from build123d import *

# Parameters (mm, degrees)
F1_DEPTH = 3
F2_DEPTH = 8
F0_W     = 2
F0_H     = 2
F3_DEPTH = 2
F4_R     = 3.6974991887
F5_DEPTH = 2


# Not quite as in the source:
# - a fillet or chamfer that OpenCascade refuses, or shapes differently, is made with other operations: its cross-section is extruded or revolved along the edge and cut away or added


with BuildPart() as f1:
    # F0 (on Top) → F1 (new body)
    with BuildSketch(Plane.XY):
        with BuildLine():
            Line((3.7669987963, -1), (3.6142080737, -1))
            ThreePointArc((3.6142080737, -1), (2.6516504294, -2.6516504294), (1, -3.6142080737))
            Line((1, -3.6142080737), (1, -5.6623758265))
            ThreePointArc((1, -5.6623758265), (4.0658639918, -4.0658639918), (5.6623758265, -1))
            Line((5.6623758265, -1), (3.7669987963, -1))
        make_face()
    extrude(amount=F1_DEPTH)



with BuildPart() as f1b:
    # F0 (on Top) → F1, piece 2 (new body)
    with BuildSketch(Plane.XY):
        with BuildLine():
            Line((-1, -5.6623758265), (-1, -3.6142080737))
            ThreePointArc((-1, -3.6142080737), (-2.6516504294, -2.6516504294), (-3.6142080737, -1))
            Line((-3.6142080737, -1), (-5.6623758265, -1))
            ThreePointArc((-5.6623758265, -1), (-4.0658639918, -4.0658639918), (-1, -5.6623758265))
        make_face()
    extrude(amount=F1_DEPTH)


with BuildPart() as f1c:
    # F0 (on Top) → F1, piece 3 (new body)
    with BuildSketch(Plane.XY):
        with BuildLine():
            ThreePointArc((-3.6142080737, 1), (-2.6516504294, 2.6516504294), (-1, 3.6142080737))
            Line((-1, 3.6142080737), (-1, 5.6623758265))
            ThreePointArc((-1, 5.6623758265), (-4.0658639918, 4.0658639918), (-5.6623758265, 1))
            Line((-5.6623758265, 1), (-3.6142080737, 1))
        make_face()
    extrude(amount=F1_DEPTH)


with BuildPart() as f1d:
    # F0 (on Top) → F1, piece 4 (new body)
    with BuildSketch(Plane.XY):
        with BuildLine():
            ThreePointArc((1, 3.6142080737), (2.6516504294, 2.6516504294), (3.6142080737, 1))
            Line((3.6142080737, 1), (5.6623758265, 1))
            ThreePointArc((5.6623758265, 1), (4.0658639918, 4.0658639918), (1, 5.6623758265))
            Line((1, 5.6623758265), (1, 3.6142080737))
        make_face()
    extrude(amount=F1_DEPTH)


with BuildPart() as f1_1:
    add(f1.part)

    add(f1b.part)  # F2 merges F1b

    add(f1c.part)  # F2 merges F1c

    add(f1d.part)  # F2 merges F1d
    # F0 (on Top) → F2 (join)
    with BuildSketch(Plane.XY):
        with BuildLine():
            ThreePointArc((0.6450651563, 3.6941021838), (0.8235020396, 3.6584620253), (1, 3.6142080737))
            Line((1, 3.6142080737), (1, 5.6623758265))
            ThreePointArc((1, 5.6623758265), (0.8229328266, 5.6908067585), (0.6450651563, 5.7137020349))
            Line((0.6450651563, 5.7137020349), (0.6450651563, 3.6941021838))
        make_face()
        with BuildLine():
            ThreePointArc((-1, 3.6142080737), (-0.8235020396, 3.6584620253), (-0.6450651563, 3.6941021838))
            Line((-0.6450651563, 3.6941021838), (-0.6450651563, 5.7137020349))
            ThreePointArc((-0.6450651563, 5.7137020349), (-0.8229328266, 5.6908067585), (-1, 5.6623758265))
            Line((-1, 5.6623758265), (-1, 3.6142080737))
        make_face()
        with BuildLine():
            ThreePointArc((-3.6142080737, -1), (-3.75, 0), (-3.6142080737, 1))
            Line((-3.6142080737, 1), (-5.6623758265, 1))
            ThreePointArc((-5.6623758265, 1), (-5.75, 0), (-5.6623758265, -1))
            Line((-5.6623758265, -1), (-3.6142080737, -1))
        make_face()
        with BuildLine():
            ThreePointArc((3.6142080737, 1), (3.7158969493, 0.5045888047), (3.75, 0))
            ThreePointArc((3.75, 0), (3.7158969493, -0.5045888047), (3.6142080737, -1))
            Line((3.6142080737, -1), (3.7669987963, -1))
            Line((3.7669987963, -1), (5.6623758265, -1))
            ThreePointArc((5.6623758265, -1), (5.7280520686, -0.5019158285), (5.75, 0))
            ThreePointArc((5.75, 0), (5.7280520686, 0.5019158285), (5.6623758265, 1))
            Line((5.6623758265, 1), (3.6142080737, 1))
        make_face()
        with BuildLine():
            Line((1, -5.6623758265), (1, -3.6142080737))
            ThreePointArc((1, -3.6142080737), (0, -3.75), (-1, -3.6142080737))
            Line((-1, -3.6142080737), (-1, -5.6623758265))
            ThreePointArc((-1, -5.6623758265), (0, -5.75), (1, -5.6623758265))
        make_face()
    extrude(amount=F2_DEPTH)

    # F0 (on Top) → F3 (join)
    with BuildSketch(Plane.XY):
        with BuildLine():
            ThreePointArc((-0.6450651563, 3.6941021838), (0, 3.75), (0.6450651563, 3.6941021838))
            Line((0.6450651563, 3.6941021838), (0.6450651563, 5.7137020349))
            ThreePointArc((0.6450651563, 5.7137020349), (0, 5.75), (-0.6450651563, 5.7137020349))
            Line((-0.6450651563, 5.7137020349), (-0.6450651563, 3.6941021838))
        make_face()
        with BuildLine():
            Line((0.6450651563, 3.1745089218), (0.6450651563, 3.6941021838))
            ThreePointArc((0.6450651563, 3.6941021838), (0, 3.75), (-0.6450651563, 3.6941021838))
            Line((-0.6450651563, 3.6941021838), (-0.6450651563, 3.1745089218))
            Line((-0.6450651563, 3.1745089218), (0.6450651563, 3.1745089218))
        make_face()
        with BuildLine():
            Line((1, 1), (1, 3.6142080737))
            ThreePointArc((1, 3.6142080737), (0.8235020396, 3.6584620253), (0.6450651563, 3.6941021838))
            Line((0.6450651563, 3.6941021838), (0.6450651563, 3.1745089218))
            Line((0.6450651563, 3.1745089218), (-0.6450651563, 3.1745089218))
            Line((-0.6450651563, 3.1745089218), (-0.6450651563, 3.6941021838))
            ThreePointArc((-0.6450651563, 3.6941021838), (-0.8235020396, 3.6584620253), (-1, 3.6142080737))
            Line((-1, 3.6142080737), (-1, 1))
            Line((-1, 1), (1, 1))
        make_face()
        with BuildLine():
            Line((-1, -1), (-1, 1))
            Line((-1, 1), (-3.6142080737, 1))
            ThreePointArc((-3.6142080737, 1), (-3.75, 0), (-3.6142080737, -1))
            Line((-3.6142080737, -1), (-1, -1))
        make_face()
        with BuildLine():
            ThreePointArc((3.6142080737, -1), (3.7158969493, -0.5045888047), (3.75, 0))
            ThreePointArc((3.75, 0), (3.7158969493, 0.5045888047), (3.6142080737, 1))
            Line((3.6142080737, 1), (1, 1))
            Line((1, 1), (1, -1))
            Line((1, -1), (3.6142080737, -1))
        make_face()
        Rectangle(F0_W, F0_H)
        with BuildLine():
            ThreePointArc((-1, -3.6142080737), (0, -3.75), (1, -3.6142080737))
            Line((1, -3.6142080737), (1, -1))
            Line((1, -1), (-1, -1))
            Line((-1, -1), (-1, -3.6142080737))
        make_face()
    extrude(amount=F3_DEPTH)

    # F4 (on face) → F5 (join)
    with BuildSketch(Plane.XY.offset(8)):
        with BuildLine():
            Line((3.6142080737, 1), (5.609054912, 1))
            ThreePointArc((5.609054912, 1), (-5.6974991887, 0), (5.609054912, -1))
            Line((5.609054912, -1), (3.6142080737, -1))
            ThreePointArc((3.6142080737, -1), (3.75, 0), (3.6142080737, 1))
        make_face()
        Circle(F4_R, mode=Mode.SUBTRACT)
    extrude(amount=-F5_DEPTH)

    # F6: fillet of radius 5 on 1 edges, made by hand

    # F6_s1 → F6_t2 (revolve, cut)
    with BuildSketch(Plane(origin=(0, 0, 0), x_dir=(0, 0, 1), z_dir=(-0.1739130435, 0.9847610133, 0))):
        with BuildLine():
            ThreePointArc((0, 0.75), (1.4644660941, 4.2855339059), (5, 5.75))
            Line((5, 5.75), (0, 5.75))
            Line((0, 5.75), (0, 0.75))
        make_face()
    revolve(axis=Axis((0, 0, 0), (0, 0, -1)), mode=Mode.SUBTRACT)


solid = f1_1.part
Here's how the part is built. I have some questions about the finished solid (model axes, mm). A direction names the side the tool comes from. Coordinates: 2 decimals unless noted, no trailing zeros. Loops run counter-clockwise (first coordinate to the right, second up) from the corner with the lowest first, then second, coordinate; pieces in that order, holes last.
1. For P1, Ø1.6, axis at x = -2, z = 1.5, coming from the -Y side; P2, Ø1, axis at y = -3.5, z = 3, coming from the -X side; P3, Ø1.5, axis at x = 2, z = 1.5, coming from the +Y side, each with a flat end and sliding along its axis, tell me the tip position at first contact or that it passes through.
2. If we mould it in two halves opening along X, with no side actions, what happens to faces 4 (the cylindrical face through (-4.063, -3.994, 7.014)), 5 (the cylindrical face through (4.063, 3.994, 7.014)), 6 (the flat face through (1, -2, 1)), 7 (the flat face through (-2, 1, 1))? For each: pulls with the +X half, pulls with the -X half, needs draft (parallel to the pull), parting line crosses it, or undercut.
3. Imagine slicing it at A-A, the plane z = 5.5. Please give me the cut outline in (x, y).
4. I need wall thicknesses on L1, parallel to Y at x = 2.75, z = 1.25; L2, parallel to X at y = 4.25, z = 5.25; L3, parallel to Z at x = 2.75, y = -4. Which ranges of each line are inside material? Lowest first, please.
5. For faces 1 (the cylindrical face through (3.527, 1.111, 7.014)), 2 (the flat face through (-3, 3, 3)), 3 (the flat face through (-3, -3, 3)), which set-ups out of +Z, -Z, +X, -X, +Y, -Y let a thin tool reach every point of the face, with its end or its side?
6. Imagine slicing it at C-C, the plane y = 1.5. Count the separate pieces of the cut face and the enclosed holes in it, and give its area (3 significant figures).
Taken from the geometry:
1. P1: stops at y = -4.62
1. P2: stops at x = -4.41
1. P3: stops at y = 4.58
2. face 4: pulls with the -X half
2. face 5: pulls with the +X half
2. face 6: undercut
2. face 7: undercut
3. outline: (-5.66, -1) - (-3.61, -1) arc R3.75 cw to (-3.61, 1) - (-5.66, 1) arc R5.75 ccw to start; (-1, -5.66) arc R5.75 ccw to (1, -5.66) - (1, -3.61) arc R3.75 cw to (-1, -3.61) - close; (-1, 3.61) arc R3.75 cw to (-0.65, 3.69) - (-0.65, 5.71) arc R5.75 ccw to (-1, 5.66) - close; (0.65, 3.69) arc R3.75 cw to (1, 3.61) - (1, 5.66) arc R5.75 ccw to (0.65, 5.71) - close; (3.61, -1) - (5.66, -1) arc R5.75 ccw to (5.66, 1) - (3.61, 1) arc R3.75 cw to start
4. L1: y = -2.98 to -2.55, -1 to 1, 2.55 to 2.98
4. L2: x = -1 to -0.65, 0.65 to 1
4. L3: z = 2.14 to 3, 6 to 8
5. face 1: +Z
5. face 2: -X, +Y
5. face 3: -X, -Y
6. separate pieces: 5
6. enclosed holes: 0
6. area: 16.3 mm2
